Can you work these out from the model? Positions are in its coordinate system, mm. A direction names the side the tool comes from. Round coordinates to 2 decimals unless told otherwise and drop trailing zeros. Loops run counter-clockwise (first coordinate to the right, second up) from the corner with the lowest first, then second, coordinate; pieces in that order, holes last. Notation, with made-up numbers: M -8,71.5 L 8,71.5 A20 cw 8,85.5 Z; hole C -26,40.25 d3. An arc over 180 degrees is marked long. Return JSON: item names as keys, results as strings.
```python
from build123d import *

# Parameters (mm, degrees)
SALIENTE_EXTRUIR2_DEPTH = 5
SALIENTE_EXTRUIR3_DEPTH = 20
REDONDEO2_R             = 5
REDONDEO3_R             = 5
CROQUIS4_R              = 60
CORTAR_EXTRUIR1_DEPTH   = 10
CROQUIS3_R              = 90
CORTAR_EXTRUIR2_DEPTH   = 3
CORTAR_EXTRUIR3_DEPTH   = 5


with BuildPart() as part:
    # Croquis1 → Saliente-Extruir2 (new body)
    with BuildSketch(Plane(origin=(0, 0, 0), x_dir=(1, 0, 0), z_dir=(0, 1, 0))):
        with BuildLine():
            Line((-119.224191345, -9.394190445), (-67.262667118, -99.394190445))
            ThreePointArc((-67.262667118, -99.394190445), (-59.942159042, -106.71469852), (-49.942159042, -109.394190445))
            Line((-49.942159042, -109.394190445), (53.980889412, -109.394190445))
            ThreePointArc((53.980889412, -109.394190445), (63.980889412, -106.71469852), (71.301397487, -99.394190445))
            Line((71.301397487, -99.394190445), (123.262921714, -9.394190445))
            ThreePointArc((123.262921714, -9.394190445), (125.942413639, 0.605809555), (123.262921714, 10.605809555))
            Line((123.262921714, 10.605809555), (71.301397487, 100.605809555))
            ThreePointArc((71.301397487, 100.605809555), (63.980889412, 107.926317631), (53.980889412, 110.605809555))
            Line((53.980889412, 110.605809555), (-49.942159042, 110.605809555))
            ThreePointArc((-49.942159042, 110.605809555), (-59.942159042, 107.926317631), (-67.262667118, 100.605809555))
            Line((-67.262667118, 100.605809555), (-119.224191345, 10.605809555))
            ThreePointArc((-119.224191345, 10.605809555), (-121.90368327, 0.605809555), (-119.224191345, -9.394190445))
        make_face()
    extrude(amount=SALIENTE_EXTRUIR2_DEPTH)

    # Croquis2 → Saliente-Extruir3 (add)
    with BuildSketch(Plane(origin=(0, 5, 0), x_dir=(1, 0, 0), z_dir=(0, 1, 0))):
        with BuildLine():
            Line((-67.262667118, 100.605809555), (-119.224191345, 10.605809555))
            ThreePointArc((-119.224191345, 10.605809555), (-121.90368327, 0.605809555), (-119.224191345, -9.394190445))
            Line((-119.224191345, -9.394190445), (-67.262667118, -99.394190445))
            ThreePointArc((-67.262667118, -99.394190445), (-59.942159042, -106.71469852), (-49.942159042, -109.394190445))
            Line((-49.942159042, -109.394190445), (53.980889412, -109.394190445))
            ThreePointArc((53.980889412, -109.394190445), (63.980889412, -106.71469852), (71.301397487, -99.394190445))
            Line((71.301397487, -99.394190445), (123.262921714, -9.394190445))
            ThreePointArc((123.262921714, -9.394190445), (125.942413639, 0.605809555), (123.262921714, 10.605809555))
            Line((123.262921714, 10.605809555), (71.301397487, 100.605809555))
            ThreePointArc((71.301397487, 100.605809555), (63.980889412, 107.926317631), (53.980889412, 110.605809555))
            Line((53.980889412, 110.605809555), (-49.942159042, 110.605809555))
            ThreePointArc((-49.942159042, 110.605809555), (-59.942159042, 107.926317631), (-67.262667118, 100.605809555))
        make_face()
        with BuildLine():
            Line((-62.932540099, 98.105809555), (-114.894064326, 8.105809555))
            ThreePointArc((-114.894064326, 8.105809555), (-116.90368327, 0.605809555), (-114.894064326, -6.894190445))
            Line((-114.894064326, -6.894190445), (-62.932540099, -96.894190445))
            ThreePointArc((-62.932540099, -96.894190445), (-57.442159042, -102.384571501), (-49.942159042, -104.394190445))
            Line((-49.942159042, -104.394190445), (53.980889412, -104.394190445))
            ThreePointArc((53.980889412, -104.394190445), (61.480889412, -102.384571501), (66.971270468, -96.894190445))
            Line((66.971270468, -96.894190445), (118.932794695, -6.894190445))
            ThreePointArc((118.932794695, -6.894190445), (120.942413639, 0.605809555), (118.932794695, 8.105809555))
            Line((118.932794695, 8.105809555), (66.971270468, 98.105809555))
            ThreePointArc((66.971270468, 98.105809555), (61.480889412, 103.596190612), (53.980889412, 105.605809555))
            Line((53.980889412, 105.605809555), (-49.942159042, 105.605809555))
            ThreePointArc((-49.942159042, 105.605809555), (-57.442159042, 103.596190612), (-62.932540099, 98.105809555))
        make_face(mode=Mode.SUBTRACT)
    extrude(amount=SALIENTE_EXTRUIR3_DEPTH)

    # Redondeo2
    redondeo2_edges = [part.edges().sort_by_distance(p)[0] for p in [
        (2.019365185, 0, -110.605809555),
        (63.980889412, 0, -107.926317631),
        (97.282159601, 0, -55.605809555),
        (125.942413639, 0, -0.605809555),
        (97.282159601, 0, 54.394190445),
        (63.980889412, 0, 106.71469852),
        (2.019365185, 0, 109.394190445),
        (-59.942159042, 0, 106.71469852),
        (-93.243429232, 0, 54.394190445),
        (-121.90368327, 0, -0.605809555),
        (-93.243429232, 0, -55.605809555),
        (-59.942159042, 0, -107.926317631),
    ]]
    fillet(redondeo2_edges, radius=REDONDEO2_R)

    # Redondeo3
    redondeo3_edges = [part.edges().sort_by_distance(p)[0] for p in [
        (-57.442159042, 5, -103.596190612),
        (-88.913302213, 5, -53.105809555),
        (-116.90368327, 5, -0.605809555),
        (-88.913302213, 5, 51.894190445),
        (-57.442159042, 5, 102.384571501),
        (2.019365185, 5, 104.394190445),
        (61.480889412, 5, 102.384571501),
        (92.952032582, 5, 51.894190445),
        (120.942413639, 5, -0.605809555),
        (92.952032582, 5, -53.105809555),
        (61.480889412, 5, -103.596190612),
        (2.019365185, 5, -105.605809555),
    ]]
    fillet(redondeo3_edges, radius=REDONDEO3_R)

    # Croquis4 → Cortar-Extruir1 (cut)
    with BuildSketch(Plane(origin=(0, 0, 0), x_dir=(-1, 0, 0), z_dir=(0, -1, 0))):
        with Locations(Location((-2.019365185, 0.605809555, 0), (0, 0, 90))):
            Circle(CROQUIS4_R)
    extrude(amount=-CORTAR_EXTRUIR1_DEPTH, mode=Mode.SUBTRACT)

    # Croquis3 → Cortar-Extruir2 (cut)
    with BuildSketch(Plane.XZ):
        with Locations(Location((2.019365185, -0.605809555, 0), (0, 0, 270))):
            Circle(CROQUIS3_R)
    extrude(amount=-CORTAR_EXTRUIR2_DEPTH, mode=Mode.SUBTRACT)

    # Croquis5 → Cortar-Extruir3 (cut)
    with BuildSketch(Plane(origin=(0, 25, 0), x_dir=(1, 0, 0), z_dir=(0, 1, 0))):
        with BuildLine():
            Line((-65.530616311, 99.605809555), (-117.492140538, 9.605809555))
            ThreePointArc((-117.492140538, 9.605809555), (-119.90368327, 0.605809555), (-117.492140538, -8.394190445))
            Line((-117.492140538, -8.394190445), (-65.530616311, -98.394190445))
            ThreePointArc((-65.530616311, -98.394190445), (-58.942159042, -104.982647713), (-49.942159042, -107.394190445))
            Line((-49.942159042, -107.394190445), (53.980889412, -107.394190445))
            ThreePointArc((53.980889412, -107.394190445), (62.980889412, -104.982647713), (69.56934668, -98.394190445))
            Line((69.56934668, -98.394190445), (121.530870907, -8.394190445))
            ThreePointArc((121.530870907, -8.394190445), (123.942413639, 0.605809555), (121.530870907, 9.605809555))
            Line((121.530870907, 9.605809555), (69.56934668, 99.605809555))
            ThreePointArc((69.56934668, 99.605809555), (62.980889412, 106.194266823), (53.980889412, 108.605809555))
            Line((53.980889412, 108.605809555), (-49.942159042, 108.605809555))
            ThreePointArc((-49.942159042, 108.605809555), (-58.942159042, 106.194266823), (-65.530616311, 99.605809555))
        make_face()
        with BuildLine():
            Line((-64.491385826, 99.005809555), (-116.452910053, 9.005809555))
            ThreePointArc((-116.452910053, 9.005809555), (-118.70368327, 0.605809555), (-116.452910053, -7.794190445))
            Line((-116.452910053, -7.794190445), (-64.491385826, -97.794190445))
            ThreePointArc((-64.491385826, -97.794190445), (-58.342159042, -103.943417228), (-49.942159042, -106.194190445))
            Line((-49.942159042, -106.194190445), (53.980889412, -106.194190445))
            ThreePointArc((53.980889412, -106.194190445), (62.380889412, -103.943417228), (68.530116195, -97.794190445))
            Line((68.530116195, -97.794190445), (120.491640422, -7.794190445))
            ThreePointArc((120.491640422, -7.794190445), (122.742413639, 0.605809555), (120.491640422, 9.005809555))
            Line((120.491640422, 9.005809555), (68.530116195, 99.005809555))
            ThreePointArc((68.530116195, 99.005809555), (62.380889412, 105.155036339), (53.980889412, 107.405809555))
            Line((53.980889412, 107.405809555), (-49.942159042, 107.405809555))
            ThreePointArc((-49.942159042, 107.405809555), (-58.342159042, 105.155036339), (-64.491385826, 99.005809555))
        make_face(mode=Mode.SUBTRACT)
    extrude(amount=-CORTAR_EXTRUIR3_DEPTH, mode=Mode.SUBTRACT)


solid = part.part
```
Q1. On a 3-axis mill with a long thin cutter (end or side, diameter ignored), from which of +Z, -Z, +X, -X, +Y, -Y can I reach the whole of each face in a straight line? I mean faces 5 (the flat face through (1, 15, 109.394)), 6 (the cylindrical face through (-57.35, 17.4, -103.65)). Say none if no direction works.
Results:
{"face 5": "+Z, +X, -X, +Y, -Y", "face 6": "+Y"}
Q2. If I drill on line 1 along Z through (x, y) = (33.5, 22.25); line 2 along Z through (x, y) = (33, 16.5); line 3 along X through (y, z) = (21.5, -37.5), over which ranges is the centre line in solid material (lowest first)?
Results:
{"line 1": "z = -110.61 to -108.61, -107.41 to -105.61, 104.39 to 106.19, 107.39 to 109.39", "line 2": "z = -110.61 to -105.61, 104.39 to 109.39", "line 3": "x = -103.7 to -101.39, -100 to -97.92, 101.96 to 104.04, 105.43 to 107.74"}
Q3. Suppose I cut it at A-A, the plane y = 14. Please give me the cut outline in (x, z).
Results:
{"outline": "M -119.22,-10.61 L -67.26,-100.61 A20 ccw -49.94,-110.61 L 53.98,-110.61 A20 ccw 71.3,-100.61 L 123.26,-10.61 A20 ccw 123.26,9.39 L 71.3,99.39 A20 ccw 53.98,109.39 L -49.94,109.39 A20 ccw -67.26,99.39 L -119.22,9.39 A20 ccw Z; hole M -114.89,-8.11 L -62.93,-98.11 A15 ccw -49.94,-105.61 L 53.98,-105.61 A15 ccw 66.97,-98.11 L 118.93,-8.11 A15 ccw 118.93,6.89 L 66.97,96.89 A15 ccw 53.98,104.39 L -49.94,104.39 A15 ccw -62.93,96.89 L -114.89,6.89 A15 ccw Z"}
Q4. I'm going to push flat-ended pins straight in: pin 1 Ø12 at (y, z) = (7, -38) entering from +X; pin 2 Ø4 at (y, z) = (5, -30) entering from +X; pin 3 Ø6 at (x, y) = (67, 14.5) entering from -Z; pin 4 Ø6 at (x, z) = (-97, -58) entering from +Y. Where does each tip first touch, or does it pass through?
Results:
{"pin 1": "stops at x = 110.91", "pin 2": "stops at x = 113.22", "pin 3": "stops at z = -107.92", "pin 4": "passes through"}
Q5. Suppose I cut it at B-B, the plane x = 43. Please give me the cut outline in (y, z), plus the area to 3 significant figures.
Results:
{"outline": "M 0,-105.61 A5 ccw 5,-110.61 L 25,-110.61 L 25,-108.61 L 20,-108.61 L 20,-107.41 L 25,-107.41 L 25,-105.61 L 10,-105.61 A5 cw 5,-100.61 L 5,-44.43 L 3,-44.43 L 3,-80.73 L 0,-80.73 Z; M 0,79.52 L 3,79.52 L 3,43.22 L 5,43.22 L 5,99.39 A5 cw 10,104.39 L 25,104.39 L 25,106.19 L 20,106.19 L 20,107.39 L 25,107.39 L 25,109.39 L 5,109.39 A5 ccw 0,104.39 Z", "area": "632 mm2"}
Q6. Thinking about a two-plate mould opening in X: for faces 1 (the cylindrical face through (1.292, 6.504, -104.18)), 2 (the cylindrical face through (125.94, 14.86, -0.46)), 3 (the cylindrical face through (-91.578, 1.426, 54.272)), 4 (the flat face through (-109, 25, -26)), which applies, pulls with the +X half, pulls with the -X half, needs draft (parallel to the pull), parting line crosses it, or undercut?
Results:
{"face 1": "undercut", "face 2": "pulls with the +X half", "face 3": "pulls with the -X half", "face 4": "needs draft"}
